Can you work these out from the model? Positions are in its coordinate system, mm. A direction names the side the tool comes from. Round coordinates to 2 decimals unless told otherwise and drop trailing zeros. Loops run counter-clockwise (first coordinate to the right, second up) from the corner with the lowest first, then second, coordinate; pieces in that order, holes last. Notation, with made-up numbers: (72, 82.25) -> (81, 82.25) arc R25 cw to (81, 121.25) -> close; hole circle Ø3 at (6, 8). An arc over 180 degrees is marked (long way). Write each question's results on one line, items separated by ' | '.
from build123d import *

# Parameters (mm, degrees)
F1_DEPTH = 50.8
F3_DEPTH = 25.4
F5_DEPTH = 10.16


with BuildPart() as f1:
    # F0 (on Front) → F1 (new body)
    with BuildSketch(Plane.XZ):
        Polygon((-72.035342, 0), (-45.047842, 0), (-22.225, 13.176774), (0, 28.575), (0, 63.5), (-120.65, 63.5), (-120.65, 28.575), (-98.425, 15.236076), align=None)
    extrude(amount=F1_DEPTH)

    # F2 (on face) → F3 (cut)
    with BuildSketch(Plane.XZ.offset(50.8)):
        Polygon((-22.225, 63.5), (-22.225, 13.176774), (0, 28.575), (0, 63.5), align=None)
        Polygon((-98.425, 15.236076), (-98.425, 63.5), (-120.65, 63.5), (-120.65, 28.575), align=None)
    extrude(amount=-F3_DEPTH, mode=Mode.SUBTRACT)

    # F4 (on face) → F5 (cut)
    with BuildSketch(Plane.YZ):
        Polygon((-22.143953, 35.172231), (-5.684754, 35.172231), (-5.684754, 38.358856), (-12.085554, 38.358856), (-12.085554, 45.369253), (-14.523953, 45.369253), (-14.523953, 38.358856), (-17.876754, 38.358856), (-17.876754, 45.369253), (-22.143953, 45.369253), align=None)
        with BuildLine():
            Line((-22.353571, 54.602597), (-22.353571, 49.187634))
            Line((-22.353571, 49.187634), (-5.304984, 49.187634))
            Line((-5.304984, 49.187634), (-5.304984, 53.145573))
            Line((-5.304984, 53.145573), (-12.81351, 53.145573))
            Line((-12.81351, 53.145573), (-5.304984, 59.421983))
            Line((-5.304984, 59.421983), (-5.304984, 62.560186))
            Line((-5.304984, 62.560186), (-12.86866, 56.237676))
            ThreePointArc((-12.86866, 56.237676), (-18.29978, 59.415003), (-22.353571, 54.602597))
        make_face()
    extrude(amount=-F5_DEPTH, mode=Mode.SUBTRACT)


solid = f1.part
1. If we section it at C-C (x = -113): List the corners of the cut face in (y, z) for me.
Final values:
outline: (-25.4, 23.98) -> (0, 23.98) -> (0, 63.5) -> (-25.4, 63.5) -> close
2. Will these pins go through, and if not, where does the flat tip stop? pin 1 (1.3 mm diameter, centred on x = -6, y = -20, fed in from -Z); pin 2 (4 mm diameter, centred on y = -29, z = 44, fed in from +X) (3 decimals); pin 3 (7.5 mm diameter, centred on x = -5.5, z = 41.5, fed in from -Y).
Final values:
pin 1: z = 23.97 | pin 2: x = -22.225 | pin 3: y = -25.4
3. If we section it at B-B (y = -41): List the corners of the cut face in (x, z) for me (3 decimals), then the cut area to 3 significant figures.
Final values:
outline: (-98.425, 15.236) -> (-72.035, 0) -> (-45.048, 0) -> (-22.225, 13.177) -> (-22.225, 63.5) -> (-98.425, 63.5) -> close | area: 4,490 mm2
4. On a 3-axis mill with a long thin cutter (end or side, diameter ignored), from which of +Z, -Z, +X, -X, +Y, -Y can I reach the whole of each face in a straight line? I mean faces 1 (the face through (-5, -9, 53.146)), 2 (the face through (-110, -25.4, 45)), 3 (the face through (-61, 0, 39)). Say none if no direction works.
Final values:
face 1: +X | face 2: +Z, -Z, -X, -Y | face 3: +Z, -Z, +X, -X, +Y
5. If we section it at D-D (z = 51): List the corners of the cut face in (x, y) for me (3 decimals), then the cut area to 3 significant figures.
Final values:
outline: (-120.65, -25.4) -> (-98.425, -25.4) -> (-98.425, -50.8) -> (-22.225, -50.8) -> (-22.225, -25.4) -> (0, -25.4) -> (0, -22.354) -> (-10.16, -22.354) -> (-10.16, -5.305) -> (0, -5.305) -> (0, 0) -> (-120.65, 0) -> close | area: 4,830 mm2
6. We'd pull the mould along Y, two halves only. Please class faces 4 (the face through (-85.41, -25.04, 7.72)), 5 (the face through (-5, -14, 35.172)), 6 (the face through (-5, -22.354, 52)), 7 (the face through (-11, -25.4, 44)): pulls with the +Y half, pulls with the -Y half, needs draft (parallel to the pull), parting line crosses it, or undercut.
Final values:
face 4: needs draft | face 5: undercut | face 6: undercut | face 7: pulls with the -Y half
7. Please list where these lines run through material, in increasing order: line 1 (Y direction, x = -9, z = 44); line 2 (Y direction, x = -100.5, z = 30.5); line 3 (X direction, y = -48, z = 16) (3 decimals). Write a range as from..to.
Final values:
line 1: -25.4..-22.14, -17.88..-14.52, -12.09..0 | line 2: -25.4..0 | line 3: -98.425..-22.225
8. If we section it at A-A (z = 41): List the corners of the cut face in (x, y) for me (3 decimals), then the cut area to 3 significant figures.
Final values:
outline: (-120.65, -25.4) -> (-98.425, -25.4) -> (-98.425, -50.8) -> (-22.225, -50.8) -> (-22.225, -25.4) -> (0, -25.4) -> (0, -22.144) -> (-10.16, -22.144) -> (-10.16, -17.877) -> (0, -17.877) -> (0, -14.524) -> (-10.16, -14.524) -> (-10.16, -12.086) -> (0, -12.086) -> (0, 0) -> (-120.65, 0) -> close | area: 4,930 mm2
